Autodesk Inventor part; units mm, degrees
ref_plane "YZ Plane" through (0, 0, 0) normal (1, 0, 0) x (0, 1, 0)
ref_plane "XZ Plane" through (0, 0, 0) normal (0, 1, 0) x (-1, 0, 0)
ref_plane "XY Plane" through (0, 0, 0) normal (0, 0, 1) x (1, 0, 0)
sketch "tabs" plane through (0, 0, 0) normal (0, 0, 1) x (1, 0, 0)
  line L0 (15.6175, 13.9118) -> (18.7675, 13.9118)
  line L1 (18.7675, 13.9118) -> (18.7675, 10.7868)
  line L2 (18.7675, 10.7868) -> (15.6175, 10.7868)
  line L3 (15.6175, 10.7868) -> (15.6175, 13.9118)
  line L4 (21.8175, 13.9118) -> (24.9675, 13.9118)
  line L5 (24.9675, 13.9118) -> (24.9675, 10.7868)
  line L6 (24.9675, 10.7868) -> (21.8175, 10.7868)
  line L7 (21.8175, 10.7868) -> (21.8175, 13.9118)
  line L8 (28.0175, 13.9118) -> (31.1675, 13.9118)
  line L9 (31.1675, 13.9118) -> (31.1675, 10.7868)
  line L10 (31.1675, 10.7868) -> (28.0175, 10.7868)
  line L11 (28.0175, 10.7868) -> (28.0175, 13.9118)
  line L12 (23.3925, 10.7868) -> (23.3925, 8.8536) construction
  point P0 (23.3925, 12.1901)
  dimension "d2" = 3.15
  dimension "d3" = 3.05
  dimension "d4" = 3.05
  dimension "d5" = 3.125
sketch "Sketch1" plane through (0, 0, 0) normal (0, 0, 1) x (1, 0, 0)
  line L0 (-25, 1.55) -> (25, 1.55)
  line L1 (25, 1.55) -> (25, -1.55)
  line L2 (25, -1.55) -> (-25, -1.55)
  line L3 (-25, -1.55) -> (-25, 1.55)
  line L4 (0, 16.9043) -> (0, -20.0235) construction
  line L5 (-32.3473, 0) -> (40.4078, 0) construction
  line L6 (-7.775, 4.675) -> (-4.625, 4.675)
  line L7 (-4.625, 4.675) -> (-4.625, 1.55)
  line L8 (-4.625, 1.55) -> (-7.775, 1.55)
  line L9 (-7.775, 1.55) -> (-7.775, 4.675)
  line L10 (-1.575, 4.675) -> (1.575, 4.675)
  line L11 (1.575, 4.675) -> (1.575, 1.55)
  line L12 (1.575, 1.55) -> (-1.575, 1.55)
  line L13 (-1.575, 1.55) -> (-1.575, 4.675)
  line L14 (4.625, 4.675) -> (7.775, 4.675)
  line L15 (7.775, 4.675) -> (7.775, 1.55)
  line L16 (7.775, 1.55) -> (4.625, 1.55)
  line L17 (4.625, 1.55) -> (4.625, 4.675)
  line L18 (0, 1.55) -> (0, -0.3832) construction
  line L19 (-7.775, -1.55) -> (-4.625, -1.55)
  line L20 (-4.625, -1.55) -> (-4.625, -4.675)
  line L21 (-4.625, -4.675) -> (-7.775, -4.675)
  line L22 (-7.775, -4.675) -> (-7.775, -1.55)
  line L23 (-1.575, -1.55) -> (1.575, -1.55)
  line L24 (1.575, -1.55) -> (1.575, -4.675)
  line L25 (1.575, -4.675) -> (-1.575, -4.675)
  line L26 (-1.575, -4.675) -> (-1.575, -1.55)
  line L27 (4.625, -1.55) -> (7.775, -1.55)
  line L28 (7.775, -1.55) -> (7.775, -4.675)
  line L29 (7.775, -4.675) -> (4.625, -4.675)
  line L30 (4.625, -4.675) -> (4.625, -1.55)
  line L31 (0, -4.675) -> (0, -6.6082) construction
  point P0 (0, 0)
  point P1 (25, 0)
  dimension "d0" = 50
  dimension "d1" = 3.1
extrude "Extrusion1" add sketch "Sketch1" along normal blind 3.1
equation "\"d2\" = mat + kerf"
equation "\"d3\" = mat - kerf"
equation "\"d4\" = mat - kerf"
equation "\"d5\" = mat + 0.5 * kerf"
equation "\"d1\" = mat"
equation "\"d6\" = mat"
properties part number "link1"
Geometry: final body of the model. Coordinates: model frame, mm. A direction names the side the tool comes from. Give positions to 0.01 mm unless a question says otherwise; leave off trailing zeros. Loops run counter-clockwise (first coordinate to the right, second up) from the corner with the lowest first, then second, coordinate; pieces in that order, holes last. Notation, with made-up numbers: (3.25, 26.5) - (45.25, 26.5) arc R19 cw to (45.25, 34.5) - close; hole circle Ø5 at (-10, -39.75). An arc over 180 degrees is marked (long way). One line per question, with ' | ' between items. Start each with the question number.
(1) Ray query, line 1 (X direction, y = 4, z = 2.4) (3 decimals); line 2 (Y direction, x = -19, z = 0.4). Return the intervals inside material, ascending. Write a range as from..to.
(2) Section query A-A on y = -3.25. Return loops of the section in (x, z) (3 decimals).
(3) Reachability of faces 1 (the flat face through (-16, -1.55, 2)), 2 (the flat face through (1.575, 3, 2)), 3 (the flat face through (-3, -1.55, 2)) from +Z, -Z, +X, -X, +Y, -Y: full face, straight path, thin tool, end or side. Return the list, or none.
(4) Section query B-B on z = 2.15. Return loops of the section in (x, y) (3 decimals).
(5) Pull-direction query (X, two-part tool) for faces 4 (the flat face through (4.625, -3, 2)), 5 (the flat face through (7.775, 3, 2)), 6 (the flat face through (6, 4.675, 2)); classes: released by +X, released by -X, zero draft, split by the parting line, or undercut.
(6) Section query C-C on x = -20. Return loops of the section in (y, z), then the cut area to 3 significant figures.
(7) Contact query for flat-ended pins moving along their axis: pin 1 (0.9 mm diameter, centred on y = 2.5, z = 1.5, fed in from +X) (3 decimals); pin 2 (1.6 mm diameter, centred on y = 3, z = 2, fed in from -X) (3 decimals); pin 3 (1.5 mm diameter, centred on x = -2.5, z = 2, fed in from -Y); pin 4 (4 mm diameter, centred on x = -12, y = -2.5, fed in from -Z). Output: stop coordinate, or through.
The answers:
1) line 1: -7.775..-4.625, -1.575..1.575, 4.625..7.775 | line 2: -1.55..1.55
2) outline: (-7.775, 0) - (-4.625, 0) - (-4.625, 3.1) - (-7.775, 3.1) - close; (-1.575, 0) - (1.575, 0) - (1.575, 3.1) - (-1.575, 3.1) - close; (4.625, 0) - (7.775, 0) - (7.775, 3.1) - (4.625, 3.1) - close
3) face 1: +Z, -Z, -X, -Y | face 2: +Z, -Z, +Y | face 3: +Z, -Z, -Y
4) outline: (-25, -1.55) - (-7.775, -1.55) - (-7.775, -4.675) - (-4.625, -4.675) - (-4.625, -1.55) - (-1.575, -1.55) - (-1.575, -4.675) - (1.575, -4.675) - (1.575, -1.55) - (4.625, -1.55) - (4.625, -4.675) - (7.775, -4.675) - (7.775, -1.55) - (25, -1.55) - (25, 1.55) - (7.775, 1.55) - (7.775, 4.675) - (4.625, 4.675) - (4.625, 1.55) - (1.575, 1.55) - (1.575, 4.675) - (-1.575, 4.675) - (-1.575, 1.55) - (-4.625, 1.55) - (-4.625, 4.675) - (-7.775, 4.675) - (-7.775, 1.55) - (-25, 1.55) - close
5) face 4: undercut | face 5: released by +X | face 6: zero draft
6) outline: (-1.55, 0) - (1.55, 0) - (1.55, 3.1) - (-1.55, 3.1) - close | area: 9.61 mm2
7) pin 1: x = 7.775 | pin 2: x = -7.775 | pin 3: y = -1.55 | pin 4: z = 0
